For this review, use the dimensioned drawing (mm, ordinates from the lowest corner) and the shaded views. A direction names the side the tool comes from. Coordinates: 2 decimals unless noted, no trailing zeros. Loops run counter-clockwise (first coordinate to the right, second up) from the corner with the lowest first, then second, coordinate; pieces in that order, holes last. Notation, with made-up numbers: M -6,22 L 42,22 A30 cw 42,61 Z; hole C -9.75,9.25 d6. An arc over 180 degrees is marked long. Write each question's results on one line, items separated by ' | '. Start each with the question number.
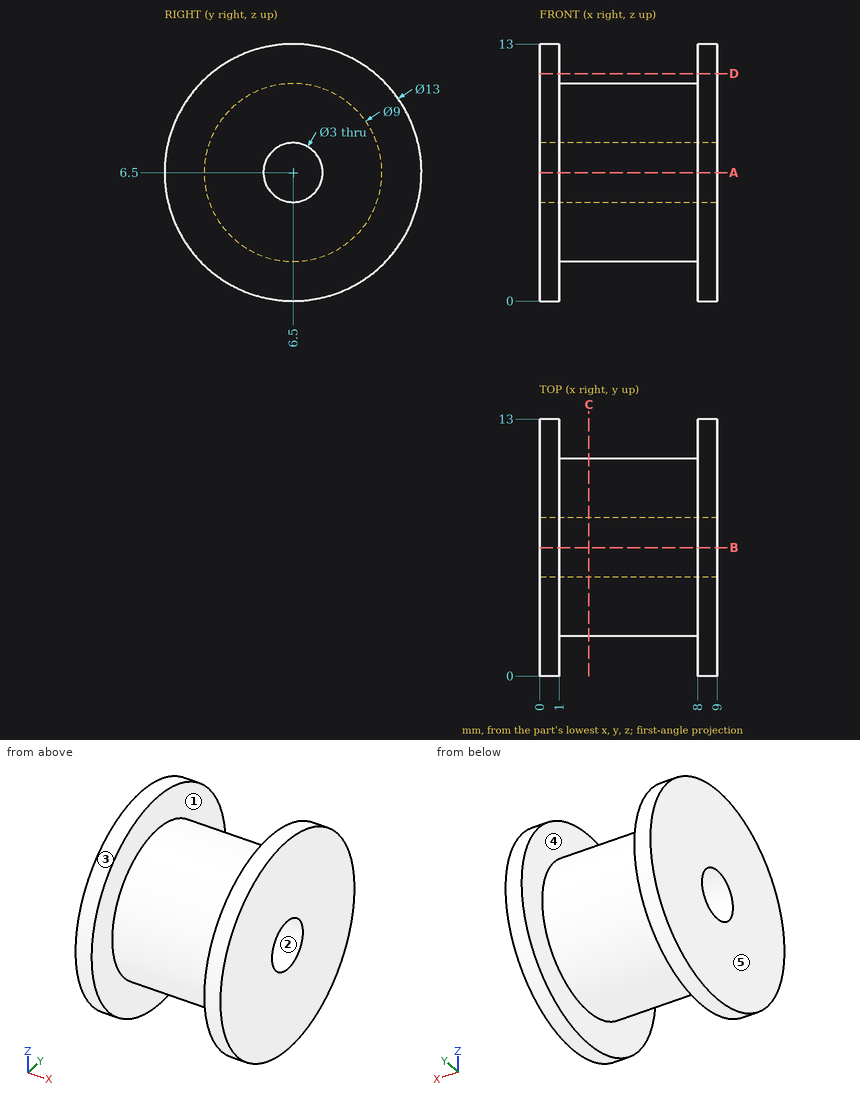
Q1. For the marked faces 4 and 5, list the 3-axis set-ups (+Z, -Z, +X, -X, +Y, -Y) from which the entire face can be reached by the end or side of a thin tool; tool diameter is ignored.
Q2. To check wall thickness, follow line 1 along X through (y, z) = (8.5, 11.75); line 2 along Y through (x, z) = (4.5, 6.5); line 3 along Z through (x, y) = (6.75, 5.75). State the ranges of each line that lie inside material, in increasing order.
Q3. The part is to be moulded in two halves that separate along Y. For the marked faces 1, 2 and 3, say which applies: pulls with the +Y half, pulls with the -Y half, needs draft (parallel to the pull), parting line crosses it, or undercut.
Q4. Insertion check: P1, Ø2, axis at x = 4.5, y = 6, coming from the +Z side; P2, Ø1, axis at x = 4.5, z = 9, coming from the +Y side; P3, Ø1.5, axis at x = 2.5, z = 5.5, coming from the +Y side. Each pin has a flat end and moves straight along its axis. Give the tip position at first contact, or say it passes through.
Q5. Take a section at C-C, the plane x = 2.5. Give the boundary of the cut face in (y, z), then the cut area to 3 significant figures.
Q6. Take a section at D-D, the plane z = 11.5. Give the boundary of the cut face in (x, y), then the cut area to 3 significant figures.
Q7. Take a section at A-A, the plane z = 6.5. Give the boundary of the cut face in (x, y), then the cut area to 3 significant figures.
Results:
1) face 4: none | face 5: +Z, -Z, -X, +Y, -Y
2) line 1: 0 to 1, 8 to 9 | line 2: 2 to 5, 8 to 11 | line 3: 2.06 to 5.2, 7.8 to 10.94
3) face 1: needs draft | face 2: undercut | face 3: parting line crosses it
4) P1: z = 11 | P2: y = 10.53 | P3: y = 10.99
5) outline: C 6.5,6.5 d9; hole C 6.5,6.5 d3 | area: 56.5 mm^2
6) outline: M 0,2.35 L 1,2.35 L 1,10.65 L 0,10.65 Z; M 8,2.35 L 9,2.35 L 9,10.65 L 8,10.65 Z | area: 16.6 mm^2
7) outline: M 0,0 L 1,0 L 1,2 L 8,2 L 8,0 L 9,0 L 9,5 L 0,5 Z; M 0,8 L 9,8 L 9,13 L 8,13 L 8,11 L 1,11 L 1,13 L 0,13 Z | area: 62.0 mm^2
